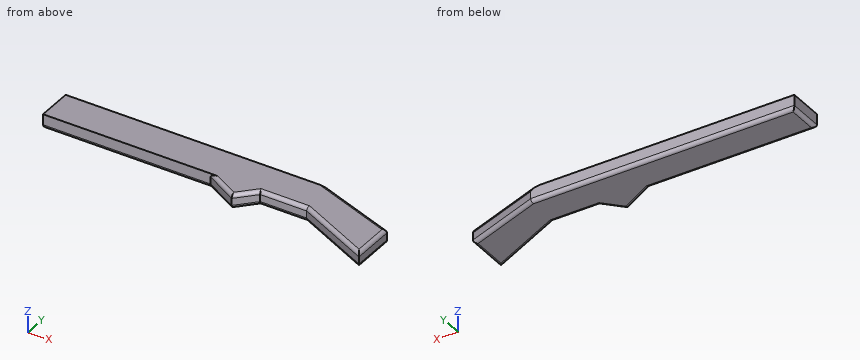
```python
from build123d import *

# Parameters (mm, degrees)
F1_DEPTH = 2
F2_R     = 0.5
F3_R     = 0.5


with BuildPart() as f1:
    # F0 (on Top) → F1 (new body)
    with BuildSketch(Plane.XY):
        Polygon((37.371002, 0), (0, 0), (0, -5), (23.76816, -5), (28.375575, -7.545115), (30.788982, -5), (37.371002, -5), (48, -10), (48, -3.815304), align=None)
    extrude(amount=F1_DEPTH)

    # F2
    f2_edges = [f1.edges().sort_by_distance(p)[0] for p in [
        (48, -6.907652, 2),
        (42.685501, -7.5, 2),
        (34.079992, -5, 2),
        (29.582279, -6.272558, 2),
        (26.071868, -6.272558, 2),
        (42.685501, -1.907652, 2),
    ]]
    fillet(f2_edges, radius=F2_R)

    # F3
    f3_edges = [f1.edges().sort_by_distance(p)[0] for p in [
        (11.88408, -5, 0),
        (26.071868, -6.272558, 0),
        (29.582279, -6.272558, 0),
        (34.079992, -5, 0),
        (42.685501, -7.5, 0),
        (18.685501, 0, 0),
        (42.685501, -1.907652, 0),
        (0, -2.5, 0),
        (48, -6.907652, 0),
    ]]
    fillet(f3_edges, radius=F3_R)


solid = f1.part
```
Geometry check sheet. Reference: the model listing, model coordinates, mm. Coordinates: 2 decimals unless noted, no trailing zeros. Write each loop counter-clockwise with the first axis right and the second up, starting at its lowest first coordinate (ties: lowest second). Pieces come first, ordered by that corner, then holes. Notation, with made-up numbers: M 7.5,21.25 L 46.5,21.25 A24 ccw 46.5,46.25 Z; hole C 56,46.25 d1. An arc over 180 degrees is marked long. Answer as a JSON object with one key per item and string values.
1. Scan lines: L1, parallel to Y at x = 33.5, z = 1.55; L2, parallel to X at y = -6, z = 0.8; L3, parallel to X at y = -7, z = 0.2. Record each from-to range of solid material in increasing order.
Answers below:
{"L1": "y = -5 to 0", "L2": "x = 25.58 to 29.84, 39.5 to 48", "L3": "x = 27.6 to 28.75, 41.86 to 47.9"}
2. Section check A-A, the plane x = 32. Enter the section's corners in (y, z).
Answers below:
{"outline": "M -5,0.5 A0.5 ccw -4.5,0 L -0.5,0 A0.5 ccw 0,0.5 L 0,2 L -4.5,2 A0.5 ccw -5,1.5 Z"}
3. Go/stop test with a flat-tipped pin: pin 1 Ø0.8 at (x, z) = (34.5, 1) entering from -Y. Record where the tip stops, or that it passes through.
Answers below:
{"pin 1": "stops at y = -5"}
4. Section check C-C, the plane x = 8. Enter the section's corners in (y, z), plus the area to 3 significant figures.
Answers below:
{"outline": "M -5,0.5 A0.5 ccw -4.5,0 L -0.5,0 A0.5 ccw 0,0.5 L 0,2 L -5,2 Z", "area": "9.89 mm²"}
5. Section check B-B, the plane z = 1.15. Enter the section's corners in (x, y).
Answers below:
{"outline": "M 0,-5 L 23.77,-5 L 28.38,-7.55 L 30.79,-5 L 37.37,-5 L 48,-10 L 48,-3.82 L 37.37,0 L 0,0 Z"}
